Can you work these out from the drawing? Everything is in mm from the part's minimum corner. Give positions to 0.01 mm unless a question says otherwise; leave off trailing zeros. Write each loop counter-clockwise with the first axis right and the second up, starting at its lowest first coordinate (ties: lowest second). Pieces come first, ordered by that corner, then holes. Notation, with made-up numbers: (-26, 32) -> (-17, 32) arc R22 cw to (-17, 54) -> close; hole circle Ø2 at (2.25, 77.25). An arc over 180 degrees is marked (long way). Return JSON: item names as keys, results as strings.
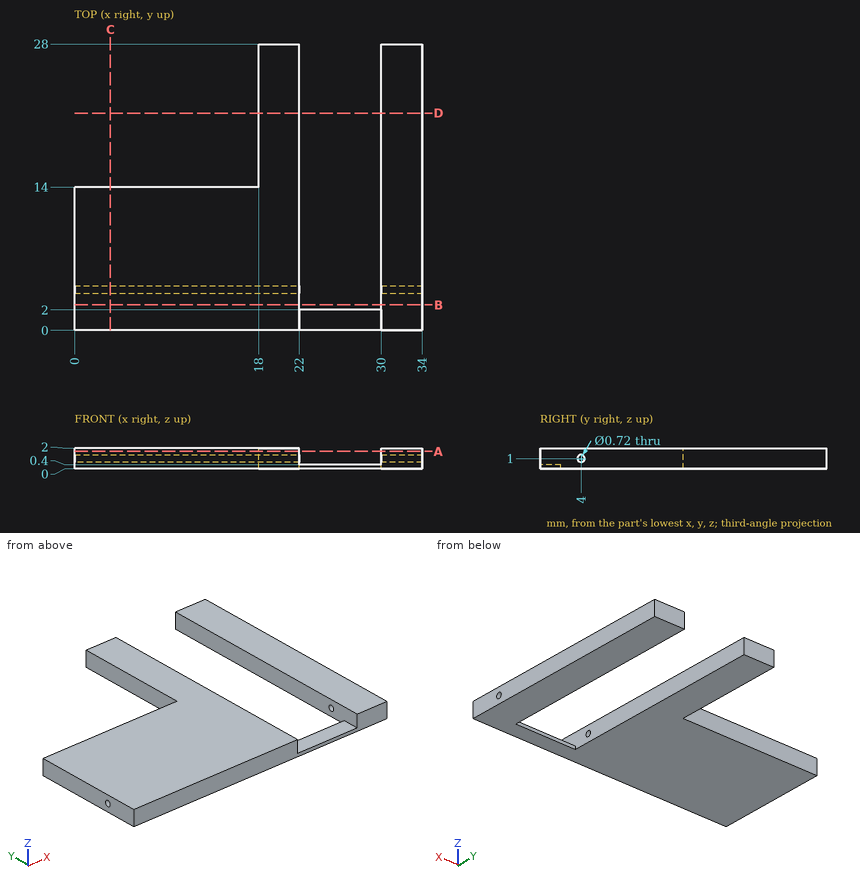
1. If I drill on line 1 (X direction, y = 17.5, z = 1.1); line 2 (Y direction, x = 11, z = 1); line 3 (X direction, y = 5, z = 1), over which ranges is the centre line in solid material (lowest first)? Write a range as [from, to].
Taken from the geometry:
{"line 1": "x = [18, 22], [30, 34]", "line 2": "y = [0, 3.64], [4.36, 14]", "line 3": "x = [0, 22], [30, 34]"}
2. Suppose I cut it at A-A, the plane z = 1.7. List the corners of the cut face in (x, y) for me.
Taken from the geometry:
{"outline": "(0, 0) -> (22, 0) -> (22, 28) -> (18, 28) -> (18, 14) -> (0, 14) -> close; (30, 0) -> (34, 0) -> (34, 28) -> (30, 28) -> close"}
3. Suppose I cut it at C-C, the plane x = 3.5. List the corners of the cut face in (y, z) for me, and give its area (3 significant figures).
Taken from the geometry:
{"outline": "(0, 0) -> (14, 0) -> (14, 2) -> (0, 2) -> close; hole circle Ø0.72 at (4, 1)", "area": "27.6 mm²"}
4. For pin 1 Ø1 at (x, y) = (24, 0.5) entering from +Z, with a flat end and sliding along its axis, tell me the tip position at first contact or that it passes through.
Taken from the geometry:
{"pin 1": "stops at z = 0.4"}
5. Suppose I cut it at B-B, the plane y = 2.5. List the corners of the cut face in (x, z) for me, and give its area (3 significant figures).
Taken from the geometry:
{"outline": "(0, 0) -> (22, 0) -> (22, 2) -> (0, 2) -> close; (30, 0) -> (34, 0) -> (34, 2) -> (30, 2) -> close", "area": "52.0 mm²"}
6. Suppose I cut it at D-D, the plane y = 21.25. List the corners of the cut face in (x, z) for me.
Taken from the geometry:
{"outline": "(18, 0) -> (22, 0) -> (22, 2) -> (18, 2) -> close; (30, 0) -> (34, 0) -> (34, 2) -> (30, 2) -> close"}
